Verification items for the finished model (mm, model axes). A direction names the side the tool comes from. Coordinates: 2 decimals unless noted, no trailing zeros. Order: outer loops, then holes, each group sorted by start corner. A loop starts at its lowest first (then second) coordinate and runs counter-clockwise, first axis right, second up. Notation, with made-up numbers: (27, 60.25) -> (73, 60.25) arc R30 cw to (73, 92.25) -> close; hole circle Ø4 at (47, 80.25). An arc over 180 degrees is marked (long way). Write item = value, one per line. Start each with the question number.
from build123d import *

# Parameters (mm, degrees)
SKETCH_1_W       = 20
SKETCH_1_H       = 10
BASEPLATE_DEPTH  = 1
HEM_OPEN_DEPTH   = 20
HEM_OPEN_2_DEPTH = 20


# Read off the part's stored shape, not the designer's step: Hem_open
# Sheet-metal steps are written as plain solids
with BuildPart() as part:
    # Sketch 1 → BasePlate (new body)
    with BuildSketch(Plane.XY):
        with Locations((10, 5)):
            Rectangle(SKETCH_1_W, SKETCH_1_H)
    extrude(amount=-BASEPLATE_DEPTH)

    # Hem_open outline → Hem_open (cut)
    with BuildSketch(Plane.YZ):
        with BuildLine():
            Line((10, 0), (9.974744871, 0))
            ThreePointArc((9.974744871, 0), (9.540569415, -0.718245837), (8.75, -1))
            Line((8.75, -1), (10, -1))
            Line((10, -1), (10, 0))
        make_face()
    extrude(amount=HEM_OPEN_DEPTH, mode=Mode.SUBTRACT)

    # Hem_open 2 outline → Hem_open 2 (add)
    with BuildSketch(Plane.YZ):
        with BuildLine():
            Line((5, 1.5), (5, 0.5))
            Line((5, 0.5), (8.75, 0.5))
            ThreePointArc((8.75, 0.5), (9, 0.25), (8.75, 0))
            Line((8.75, 0), (9.974744871, 0))
            ThreePointArc((9.974744871, 0), (9.718245837, 1.040569415), (8.75, 1.5))
            Line((8.75, 1.5), (5, 1.5))
        make_face()
    extrude(amount=HEM_OPEN_2_DEPTH)


solid = part.part
Item 1: Section check A-A (y = 8.25). Record the boundary of the cut face in (x, z).
Item 2: Thickness scan on line 1 (Z direction, x = 3, y = 6); line 2 (Y direction, x = 14.5, z = 0.3); line 3 (Z direction, x = 5.75, y = 4.5). Record the ranges inside material, lowest first.
Item 3: Section check B-B (x = 12). Record the boundary of the cut face in (y, z).
Item 4: Mould release check, pull along Z, two halves, no side actions. Record for faces 1 (the flat face through (10, 4, -1)), 2 (the flat face through (10, 7, 1.5)), 3 (the flat face through (10, 7, 0.5)), 4 (the flat face through (9.9, 0, -0.5)): pulls with the +Z half, pulls with the -Z half, needs draft (parallel to the pull), parting line crosses it, or undercut.
Item 5: Section check C-C (z = 0.25). Record the boundary of the cut face in (x, y), then the cut area to 3 significant figures.
Item 6: Tool access check on faces 5 (the flat face through (0, 6, -0.3)), 6 (the flat face through (10, 4, 0)), 7 (the flat face through (10, 5, 1)). Record the directions out of +Z, -Z, +X, -X, +Y, -Y that give a thin tool (end or side, any length) a straight path to the whole face; none if there is none.
Item 7: Gauge pin test, flat end, axial feed: P1, Ø1.5, axis at x = 10, z = 0, coming from the +Y side. Record the tip position at first contact, or that the pin passes through.
Item 8: Section check D-D (y = 1). Record the boundary of the cut face in (x, z).
Filled sheet:
q1.outline = (0, -1) -> (20, -1) -> (20, 0) -> (0, 0) -> close; (0, 0.5) -> (20, 0.5) -> (20, 1.5) -> (0, 1.5) -> close
q2.line_1 = -1 to 0, 0.5 to 1.5
q2.line_2 = 8.99 to 10
q2.line_3 = -1 to 0
q3.outline = (0, -1) -> (8.75, -1) arc R1.25 ccw to (8.75, 1.5) -> (5, 1.5) -> (5, 0.5) -> (8.75, 0.5) arc R0.25 cw to (8.75, 0) -> (0, 0) -> close
q4.face_1 = pulls with the -Z half
q4.face_2 = pulls with the +Z half
q4.face_3 = undercut
q4.face_4 = needs draft
q5.outline = (0, 9) -> (20, 9) -> (20, 10) -> (0, 10) -> close
q5.area = 20.0 mm^2
q6.face_5 = +Z, -Z, -X, +Y, -Y
q6.face_6 = +X, -X, -Y
q6.face_7 = +Z, +X, -X, -Y
q7.P1 = 10
q8.outline = (0, -1) -> (20, -1) -> (20, 0) -> (0, 0) -> close
